Geometry: final body of the model. Coordinates: model frame, mm. A direction names the side the tool comes from. Give positions to 0.01 mm unless a question says otherwise; leave off trailing zeros. Write each loop counter-clockwise with the first axis right and the second up, starting at its lowest first coordinate (ties: lowest second). Pieces come first, ordered by that corner, then holes.
```python
from build123d import *

# Parameters (mm, degrees)
SM_BASE_FLANGE_1_DEPTH            = 5
SM_EDGE_FLANGE_1_STRIP_W          = 26
SM_EDGE_FLANGE_1_STRIP_H          = 5
SM_EDGE_FLANGE_1_STRIP_CUT_DEPTH  = 45
SM_EDGE_FLANGE_1_RELIEF_W         = 28.5
SM_EDGE_FLANGE_1_RELIEF_H         = 2.5
SM_EDGE_FLANGE_1_RELIEF_CUT_DEPTH = 5
SM_EDGE_FLANGE_1_DEPTH            = 45
SM_EDGE_FLANGE_2_STRIP_W          = 26
SM_EDGE_FLANGE_2_STRIP_H          = 5
SM_EDGE_FLANGE_2_STRIP_CUT_DEPTH  = 45
SM_EDGE_FLANGE_2_RELIEF_W         = 28.5
SM_EDGE_FLANGE_2_RELIEF_H         = 2.5
SM_EDGE_FLANGE_2_RELIEF_CUT_DEPTH = 5
SM_EDGE_FLANGE_2_DEPTH            = 45
SM_EDGE_FLANGE_14_DEPTH           = 40
SM_EDGE_FLANGE_15_DEPTH           = 40
SM_EDGE_FLANGE_16_DEPTH           = 40
SM_EDGE_FLANGE_17_DEPTH           = 40
SM_EDGE_FLANGE_18_STRIP_W         = 26
SM_EDGE_FLANGE_18_STRIP_H         = 5
SM_EDGE_FLANGE_18_STRIP_CUT_DEPTH = 40
SM_EDGE_FLANGE_18_DEPTH           = 40
SM_EDGE_FLANGE_19_STRIP_W         = 26
SM_EDGE_FLANGE_19_STRIP_H         = 5
SM_EDGE_FLANGE_19_STRIP_CUT_DEPTH = 40
SM_EDGE_FLANGE_19_DEPTH           = 40
SM_EDGE_FLANGE_20_STRIP_W         = 26
SM_EDGE_FLANGE_20_STRIP_H         = 5
SM_EDGE_FLANGE_20_STRIP_CUT_DEPTH = 40
SM_EDGE_FLANGE_20_DEPTH           = 40
SM_EDGE_FLANGE_21_STRIP_W         = 26
SM_EDGE_FLANGE_21_STRIP_H         = 5
SM_EDGE_FLANGE_21_STRIP_CUT_DEPTH = 40
SM_EDGE_FLANGE_21_DEPTH           = 40
CUT_EXTRUDE_START                 = -25
SKETCH_80_R                       = 2.5
CUT_EXTRUDE_1_DEPTH               = 5
CUT_EXTRUDE_3_DEPTH               = 124.060960503
CUT_EXTRUDE_3_DEPTH_BACK          = 124.060960503
SKETCH_83_R                       = 2.5
CUT_EXTRUDE_START_2               = -20
SKETCH_84_R                       = 2.5
CUT_EXTRUDE_5_DEPTH               = 5


# Sheet-metal steps are written as plain solids
with BuildPart() as part:
    # Sketch 1 → 基体-法兰1 (new body)
    with BuildSketch(Plane(origin=(0, 0, 0), x_dir=(1, 0, 0), z_dir=(0, 1, 0))):
        Polygon((-25, -25), (-25, -50), (-50, -50), (-50, 50), (-25, 50), (-25, 25), (25, 25), (25, 50), (50, 50), (50, -50), (25, -50), (25, -25), align=None)
    extrude(amount=-SM_BASE_FLANGE_1_DEPTH)

    # 边线-法兰1 strip (across the edge) → 边线-法兰1 strip cut (cut)
    with BuildSketch(Plane(origin=(22.5, 0, -25), x_dir=(0, 0, 1), z_dir=(-1, 0, 0))):
        with Locations((-10, -2.5)):
            Rectangle(SM_EDGE_FLANGE_1_STRIP_W, SM_EDGE_FLANGE_1_STRIP_H)
    extrude(amount=SM_EDGE_FLANGE_1_STRIP_CUT_DEPTH, mode=Mode.SUBTRACT)

    # 边线-法兰1 relief (on the sheet) → 边线-法兰1 relief cut (cut)
    with BuildSketch(Plane(origin=(22.5, 0, -22), x_dir=(0, 0, 1), z_dir=(0, 1, 0))):
        with Locations((-11.75, 1.25)):
            Rectangle(SM_EDGE_FLANGE_1_RELIEF_W, SM_EDGE_FLANGE_1_RELIEF_H)
        with Locations((-11.75, -46.25)):
            Rectangle(SM_EDGE_FLANGE_1_RELIEF_W, SM_EDGE_FLANGE_1_RELIEF_H)
    extrude(amount=-SM_EDGE_FLANGE_1_RELIEF_CUT_DEPTH, mode=Mode.SUBTRACT)

    # 边线-法兰1 section (across the edge) → 边线-法兰1 (add)
    with BuildSketch(Plane(origin=(22.5, 0, -25), x_dir=(0, 0, 1), z_dir=(-1, 0, 0))):
        with BuildLine():
            Line((-5, 3), (-5, 70))
            Line((-5, 70), (0, 70))
            Line((0, 70), (0, 3))
            ThreePointArc((0, 3), (0.878679656, 0.878679656), (3, 0))
            Line((3, 0), (3, -5))
            ThreePointArc((3, -5), (-2.656854249, -2.656854249), (-5, 3))
        make_face()
    extrude(amount=SM_EDGE_FLANGE_1_DEPTH)

    # 边线-法兰2 strip (across the edge) → 边线-法兰2 strip cut (cut)
    with BuildSketch(Plane(origin=(-22.5, 0, 25), x_dir=(0, 0, -1), z_dir=(1, 0, 0))):
        with Locations((-10, -2.5)):
            Rectangle(SM_EDGE_FLANGE_2_STRIP_W, SM_EDGE_FLANGE_2_STRIP_H)
    extrude(amount=SM_EDGE_FLANGE_2_STRIP_CUT_DEPTH, mode=Mode.SUBTRACT)

    # 边线-法兰2 relief (on the sheet) → 边线-法兰2 relief cut (cut)
    with BuildSketch(Plane(origin=(-22.5, 0, 22), x_dir=(0, 0, -1), z_dir=(0, 1, 0))):
        with Locations((-11.75, 1.25)):
            Rectangle(SM_EDGE_FLANGE_2_RELIEF_W, SM_EDGE_FLANGE_2_RELIEF_H)
        with Locations((-11.75, -46.25)):
            Rectangle(SM_EDGE_FLANGE_2_RELIEF_W, SM_EDGE_FLANGE_2_RELIEF_H)
    extrude(amount=-SM_EDGE_FLANGE_2_RELIEF_CUT_DEPTH, mode=Mode.SUBTRACT)

    # 边线-法兰2 section (across the edge) → 边线-法兰2 (add)
    with BuildSketch(Plane(origin=(-22.5, 0, 25), x_dir=(0, 0, -1), z_dir=(1, 0, 0))):
        with BuildLine():
            Line((-5, 3), (-5, 70))
            Line((-5, 70), (0, 70))
            Line((0, 70), (0, 3))
            ThreePointArc((0, 3), (0.878679656, 0.878679656), (3, 0))
            Line((3, 0), (3, -5))
            ThreePointArc((3, -5), (-2.656854249, -2.656854249), (-5, 3))
        make_face()
    extrude(amount=SM_EDGE_FLANGE_2_DEPTH)

    # 边线-法兰14 section (across the edge) → 边线-法兰14 (add)
    with BuildSketch(Plane(origin=(53, -5, 10), x_dir=(-1, 0, 0), z_dir=(0, 0, 1))):
        with BuildLine():
            Line((-5, 3), (-5, 20))
            Line((-5, 20), (0, 20))
            Line((0, 20), (0, 3))
            ThreePointArc((0, 3), (0.878679656, 0.878679656), (3, 0))
            Line((3, 0), (3, -5))
            ThreePointArc((3, -5), (-2.656854249, -2.656854249), (-5, 3))
        make_face()
    extrude(amount=SM_EDGE_FLANGE_14_DEPTH)

    # 边线-法兰15 section (across the edge) → 边线-法兰15 (add)
    with BuildSketch(Plane(origin=(53, -5, -50), x_dir=(-1, 0, 0), z_dir=(0, 0, 1))):
        with BuildLine():
            Line((-5, 3), (-5, 20))
            Line((-5, 20), (0, 20))
            Line((0, 20), (0, 3))
            ThreePointArc((0, 3), (0.878679656, 0.878679656), (3, 0))
            Line((3, 0), (3, -5))
            ThreePointArc((3, -5), (-2.656854249, -2.656854249), (-5, 3))
        make_face()
    extrude(amount=SM_EDGE_FLANGE_15_DEPTH)

    # 边线-法兰16 section (across the edge) → 边线-法兰16 (add)
    with BuildSketch(Plane(origin=(-53, -5, -10), x_dir=(1, 0, 0), z_dir=(0, 0, -1))):
        with BuildLine():
            Line((-5, 3), (-5, 20))
            Line((-5, 20), (0, 20))
            Line((0, 20), (0, 3))
            ThreePointArc((0, 3), (0.878679656, 0.878679656), (3, 0))
            Line((3, 0), (3, -5))
            ThreePointArc((3, -5), (-2.656854249, -2.656854249), (-5, 3))
        make_face()
    extrude(amount=SM_EDGE_FLANGE_16_DEPTH)

    # 边线-法兰17 section (across the edge) → 边线-法兰17 (add)
    with BuildSketch(Plane(origin=(-53, -5, 50), x_dir=(1, 0, 0), z_dir=(0, 0, -1))):
        with BuildLine():
            Line((-5, 3), (-5, 20))
            Line((-5, 20), (0, 20))
            Line((0, 20), (0, 3))
            ThreePointArc((0, 3), (0.878679656, 0.878679656), (3, 0))
            Line((3, 0), (3, -5))
            ThreePointArc((3, -5), (-2.656854249, -2.656854249), (-5, 3))
        make_face()
    extrude(amount=SM_EDGE_FLANGE_17_DEPTH)

    # 边线-法兰18 strip (across the edge) → 边线-法兰18 strip cut (cut)
    with BuildSketch(Plane(origin=(-58, -25, -50), x_dir=(0, 1, 0), z_dir=(0, 0, 1))):
        with Locations((-5, -2.5)):
            Rectangle(SM_EDGE_FLANGE_18_STRIP_W, SM_EDGE_FLANGE_18_STRIP_H)
    extrude(amount=SM_EDGE_FLANGE_18_STRIP_CUT_DEPTH, mode=Mode.SUBTRACT)

    # 边线-法兰18 section (across the edge) → 边线-法兰18 (add)
    with BuildSketch(Plane(origin=(-58, -25, -50), x_dir=(0, 1, 0), z_dir=(0, 0, 1))):
        with BuildLine():
            Line((0, 3), (0, 30))
            Line((0, 30), (5, 30))
            Line((5, 30), (5, 3))
            ThreePointArc((5, 3), (5.878679656, 0.878679656), (8, 0))
            Line((8, 0), (8, -5))
            ThreePointArc((8, -5), (2.343145751, -2.656854249), (0, 3))
        make_face()
    extrude(amount=SM_EDGE_FLANGE_18_DEPTH)

    # 边线-法兰19 strip (across the edge) → 边线-法兰19 strip cut (cut)
    with BuildSketch(Plane(origin=(-58, -25, 10), x_dir=(0, 1, 0), z_dir=(0, 0, 1))):
        with Locations((-5, -2.5)):
            Rectangle(SM_EDGE_FLANGE_19_STRIP_W, SM_EDGE_FLANGE_19_STRIP_H)
    extrude(amount=SM_EDGE_FLANGE_19_STRIP_CUT_DEPTH, mode=Mode.SUBTRACT)

    # 边线-法兰19 section (across the edge) → 边线-法兰19 (add)
    with BuildSketch(Plane(origin=(-58, -25, 10), x_dir=(0, 1, 0), z_dir=(0, 0, 1))):
        with BuildLine():
            Line((0, 3), (0, 30))
            Line((0, 30), (5, 30))
            Line((5, 30), (5, 3))
            ThreePointArc((5, 3), (5.878679656, 0.878679656), (8, 0))
            Line((8, 0), (8, -5))
            ThreePointArc((8, -5), (2.343145751, -2.656854249), (0, 3))
        make_face()
    extrude(amount=SM_EDGE_FLANGE_19_DEPTH)

    # 边线-法兰20 strip (across the edge) → 边线-法兰20 strip cut (cut)
    with BuildSketch(Plane(origin=(58, -25, 50), x_dir=(0, 1, 0), z_dir=(0, 0, -1))):
        with Locations((-5, -2.5)):
            Rectangle(SM_EDGE_FLANGE_20_STRIP_W, SM_EDGE_FLANGE_20_STRIP_H)
    extrude(amount=SM_EDGE_FLANGE_20_STRIP_CUT_DEPTH, mode=Mode.SUBTRACT)

    # 边线-法兰20 section (across the edge) → 边线-法兰20 (add)
    with BuildSketch(Plane(origin=(58, -25, 50), x_dir=(0, 1, 0), z_dir=(0, 0, -1))):
        with BuildLine():
            Line((0, 3), (0, 30))
            Line((0, 30), (5, 30))
            Line((5, 30), (5, 3))
            ThreePointArc((5, 3), (5.878679656, 0.878679656), (8, 0))
            Line((8, 0), (8, -5))
            ThreePointArc((8, -5), (2.343145751, -2.656854249), (0, 3))
        make_face()
    extrude(amount=SM_EDGE_FLANGE_20_DEPTH)

    # 边线-法兰21 strip (across the edge) → 边线-法兰21 strip cut (cut)
    with BuildSketch(Plane(origin=(58, -25, -10), x_dir=(0, 1, 0), z_dir=(0, 0, -1))):
        with Locations((-5, -2.5)):
            Rectangle(SM_EDGE_FLANGE_21_STRIP_W, SM_EDGE_FLANGE_21_STRIP_H)
    extrude(amount=SM_EDGE_FLANGE_21_STRIP_CUT_DEPTH, mode=Mode.SUBTRACT)

    # 边线-法兰21 section (across the edge) → 边线-法兰21 (add)
    with BuildSketch(Plane(origin=(58, -25, -10), x_dir=(0, 1, 0), z_dir=(0, 0, -1))):
        with BuildLine():
            Line((0, 3), (0, 30))
            Line((0, 30), (5, 30))
            Line((5, 30), (5, 3))
            ThreePointArc((5, 3), (5.878679656, 0.878679656), (8, 0))
            Line((8, 0), (8, -5))
            ThreePointArc((8, -5), (2.343145751, -2.656854249), (0, 3))
        make_face()
    extrude(amount=SM_EDGE_FLANGE_21_DEPTH)

    # 草图80 → 切除-拉伸1 (cut)
    with BuildSketch(Plane(origin=(0, 0, 0), x_dir=(1, 0, 0), z_dir=(0, 1, 0)).offset(CUT_EXTRUDE_START)):
        with Locations(Location((-75, 40, 0), (0, 0, 270))):
            Circle(SKETCH_80_R)
        with Locations(Location((75, 40, 0), (0, 0, 270))):
            Circle(SKETCH_80_R)
        with Locations(Location((-75, -40, 0), (0, 0, 270))):
            Circle(SKETCH_80_R)
        with Locations(Location((75, -40, 0), (0, 0, 270))):
            Circle(SKETCH_80_R)
    extrude(amount=CUT_EXTRUDE_1_DEPTH, mode=Mode.SUBTRACT)

    # 草图83 → 切除-拉伸3 (cut, two sides: drawn at the far end of the back side and taken through both)
    with BuildSketch(Plane.XY.offset(-CUT_EXTRUDE_3_DEPTH_BACK)):
        with Locations((0, 50)):
            Circle(SKETCH_83_R)
        with Locations((0, 30)):
            Circle(SKETCH_83_R)
    extrude(amount=CUT_EXTRUDE_3_DEPTH + CUT_EXTRUDE_3_DEPTH_BACK, mode=Mode.SUBTRACT)

    # 草图84 → 切除-拉伸5 (cut)
    with BuildSketch(Plane(origin=(0, 0, 0), x_dir=(1, 0, 0), z_dir=(0, 1, 0)).offset(CUT_EXTRUDE_START_2)):
        with Locations(Location((75, 22.5, 0), (0, 0, 270))):
            Circle(SKETCH_84_R)
        with Locations(Location((75, -22.5, 0), (0, 0, 270))):
            Circle(SKETCH_84_R)
        with Locations(Location((-75, -22.5, 0), (0, 0, 270))):
            Circle(SKETCH_84_R)
        with Locations(Location((-75, 22.5, 0), (0, 0, 270))):
            Circle(SKETCH_84_R)
    extrude(amount=-CUT_EXTRUDE_5_DEPTH, mode=Mode.SUBTRACT)


solid = part.part
```
Item 1: Reachability of faces 1 (the face through (0.315, -2.719, -27.594)), 2 (the face through (53, -13, 30)), 3 (the face through (-25, -2, 35)), 4 (the face through (58, -12, 30)) from +Z, -Z, +X, -X, +Y, -Y: full face, straight path, thin tool, end or side. Return the list, or none.
Found:
face 1: -Z, -Y
face 2: +Z, -Z, -Y
face 3: +Z, +Y, -Y
face 4: +Z, -Z, +X, +Y
Item 2: Line query: L1, parallel to X at y = -23.8, z = -40; L2, parallel to Y at x = 0, z = 28; L3, parallel to Y at x = 0, z = 26.05. Output: solid intervals per line, ascending.
Found:
L1: x = -88 to -77.5, -72.5 to -56.79, 56.79 to 72.5, 77.5 to 88
L2: y = -2.29 to 27.5, 32.5 to 47.5, 52.5 to 70
L3: y = -3.9 to 27.5, 32.5 to 47.5, 52.5 to 70
Item 3: Section D-D, the plane x = 75. Return the cut outline in (y, z), plus the area to 3 significant figures.
Found:
outline: (-25, -50) - (-20, -50) - (-20, -42.5) - (-25, -42.5) - close; (-25, -37.5) - (-20, -37.5) - (-20, -25) - (-25, -25) - close; (-25, -20) - (-20, -20) - (-20, -10) - (-25, -10) - close; (-25, 10) - (-20, 10) - (-20, 20) - (-25, 20) - close; (-25, 25) - (-20, 25) - (-20, 37.5) - (-25, 37.5) - close; (-25, 42.5) - (-20, 42.5) - (-20, 50) - (-25, 50) - close
area: 300 mm2
Item 4: Section A-A, the plane y = 57. Return the cut outline in (x, z).
Found:
outline: (-22.5, -30) - (22.5, -30) - (22.5, -25) - (-22.5, -25) - close; (-22.5, 25) - (22.5, 25) - (22.5, 30) - (-22.5, 30) - close
Item 5: Pin query (flat end, axial travel): pin 1 Ø6.5 at (x, z) = (-75, -40) entering from -Y; pin 2 Ø10 at (y, z) = (29, 30) entering from -X; pin 3 Ø12 at (x, z) = (-10.5, -21) entering from -Y; pin 4 Ø13.5 at (x, y) = (10, 49.5) entering from +Z. Return the tip coordinate at first contact, or that it passes through.
Found:
pin 1: stops at y = -25
pin 2: stops at x = -22.5
pin 3: stops at y = -5
pin 4: stops at z = 30
Item 6: Pull-direction query (X, two-part tool) for faces 5 (the face through (0, 37, -25)), 6 (the face through (-0.54, 47.56, -27.53)), 7 (the face through (88, -23, -30)); classes: +X half, -X half, draft (parallel to the pull), parting line (faces both ways), or undercut.
Found:
face 5: draft
face 6: undercut
face 7: +X half
Item 7: Section B-B, the plane x = 0. Return the cut outline in (y, z).
Found:
outline: (-5, -22) arc R8 ccw to (3, -30) - (27.5, -30) - (27.5, -25) - (3, -25) arc R3 cw to (0, -22) - (0, 22) arc R3 cw to (3, 25) - (27.5, 25) - (27.5, 30) - (3, 30) arc R8 ccw to (-5, 22) - close; (32.5, -30) - (47.5, -30) - (47.5, -25) - (32.5, -25) - close; (32.5, 25) - (47.5, 25) - (47.5, 30) - (32.5, 30) - close; (52.5, -30) - (70, -30) - (70, -25) - (52.5, -25) - close; (52.5, 25) - (70, 25) - (70, 30) - (52.5, 30) - close
Item 8: Section C-C, the plane y = 30. Return the cut outline in (x, z).
Found:
outline: (-22.5, -30) - (-2.5, -30) - (-2.5, -25) - (-22.5, -25) - close; (-22.5, 25) - (-2.5, 25) - (-2.5, 30) - (-22.5, 30) - close; (2.5, -30) - (22.5, -30) - (22.5, -25) - (2.5, -25) - close; (2.5, 25) - (22.5, 25) - (22.5, 30) - (2.5, 30) - close
